Design review of the part shown in the three views and the two pictorial views. Dimensions are in mm from the part's minimum x, y and z. Give positions to 0.01 mm unless a question says otherwise; leave off trailing zeros. Order: outer loops, then holes, each group sorted by start corner. A loop starts at its lowest first (then second) coordinate and runs counter-clockwise, first axis right, second up. Notation, with made-up numbers: (23.25, 62.5) - (66.25, 62.5) arc R16 ccw to (66.25, 89.5) - close; hole circle Ø8 at (82, -15.75). An arc over 180 degrees is marked (long way). Put each result on its own line as item: value.
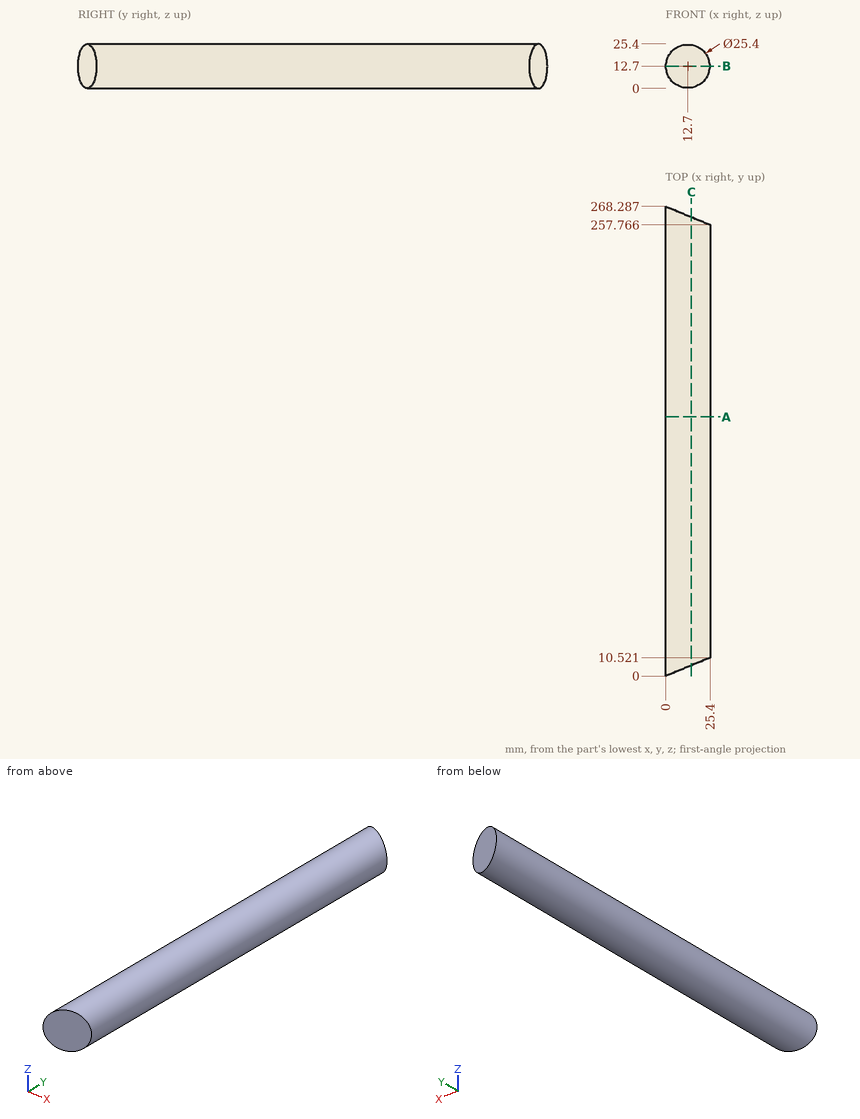
(1) Take a section at B-B, the plane z = 12.7. Write out the cut boundary in (x, y).
The answers:
outline: (0, 0) - (25.4, 10.52) - (25.4, 257.77) - (0, 268.29) - close
(2) Clearance check with flat-ended pins moving along their axes: pin 1 Ø8 at (x, y) = (2.5, 71.5) entering from +Z; pin 2 Ø4 at (x, y) = (22.5, 54.5) entering from +Z; pin 3 Ø6 at (x, z) = (18, 10) entering from -Y. State where each tip first meets the part, or that it passes through.
The answers:
pin 1: z = 23.78
pin 2: z = 22.72
pin 3: y = 6.21
(3) Take a section at A-A, the plane y = 148. Write out the cut boundary in (x, z), then the cut area to 3 significant figures.
The answers:
outline: circle Ø25.4 at (12.7, 12.7)
area: 507 mm^2
(4) Wall thickness on L1, parallel to X at y = 219, z = 13.75; L2, parallel to X at y = 153, z = 21; L3, parallel to Y at x = 7.25, z = 1.5 (1 decimal): over which ranges is each line inside the solid? List them lowest first.
The answers:
L1: 0.04 to 25.36
L2: 3.09 to 22.31
L3: 3 to 265.3
(5) Take a section at C-C, the plane x = 14.75. Write out the cut boundary in (y, z).
The answers:
outline: (6.11, 0.17) - (262.18, 0.17) - (262.18, 25.23) - (6.11, 25.23) - close
